The model under review builds one solid part; all positions refer to its coordinate system, in mm. A direction names the side the tool comes from. Give positions to 0.01 mm unless a question says otherwise; leave off trailing zeros. Write each loop counter-clockwise with the first axis right and the second up, starting at its lowest first coordinate (ties: lowest second). Pieces come first, ordered by that corner, then holes. Notation, with made-up numbers: M 83.25,-18.75 L 99.25,-18.75 A37 ccw 99.25,17.25 Z; hole C 21,63.25 d7. An arc over 180 degrees is marked long. Write each question's results on one line, items separated by ' | '. Start each with the question number.
from build123d import *

# Parameters (mm, degrees)
CROQUIS1_W                 = 2.5
CROQUIS1_H                 = 13.5
SALIENTE_EXTRUIR1_DEPTH    = 4.5
CORTAR_EXTRUIR4_DEPTH      = 10
CORTAR_EXTRUIR4_DEPTH_BACK = 23.169799277
CROQUIS7_R                 = 1.125
REDONDEO3_R                = 1


with BuildPart() as part:
    # Croquis1 → Saliente-Extruir1 (new body)
    with BuildSketch(Plane(origin=(0, 0, 0), x_dir=(1, 0, 0), z_dir=(0, 1, 0))):
        with BuildLine():
            Line((-2, -10), (2, -10))
            ThreePointArc((2, -10), (4.121320344, -9.121320344), (5, -7))
            Line((5, -7), (11, -7))
            Line((11, -7), (11, -3))
            Line((11, -3), (5, -3))
            Line((5, -3), (5, 3))
            Line((5, 3), (11, 3))
            Line((11, 3), (11, 7))
            Line((11, 7), (5, 7))
            ThreePointArc((5, 7), (4.121320344, 9.121320344), (2, 10))
            Line((2, 10), (-2, 10))
            ThreePointArc((-2, 10), (-4.121320344, 9.121320344), (-5, 7))
            Line((-5, 7), (-17, 7))
            Line((-17, 7), (-17, 3))
            Line((-17, 3), (-5, 3))
            Line((-5, 3), (-5, -3))
            Line((-5, -3), (-17, -3))
            Line((-17, -3), (-17, -7))
            Line((-17, -7), (-5, -7))
            ThreePointArc((-5, -7), (-4.121320344, -9.121320344), (-2, -10))
        make_face()
        Rectangle(CROQUIS1_W, CROQUIS1_H, mode=Mode.SUBTRACT)
    extrude(amount=SALIENTE_EXTRUIR1_DEPTH)

    # Croquis7 → Cortar-Extruir4 (cut, two sides: drawn at the far end of the back side and taken through both)
    with BuildSketch(Plane.XY.offset(3.5).offset(-CORTAR_EXTRUIR4_DEPTH_BACK)):
        with Locations(Location((-14.5, 2.25, 0), (0, 0, 180))):
            Circle(CROQUIS7_R)
        with Locations(Location((8.5, 2.25, 0), (0, 0, 180))):
            Circle(CROQUIS7_R)
        with Locations(Location((-7.5, 2.25, 0), (0, 0, 180))):
            Circle(CROQUIS7_R)
    extrude(amount=CORTAR_EXTRUIR4_DEPTH + CORTAR_EXTRUIR4_DEPTH_BACK, mode=Mode.SUBTRACT)

    # Redondeo3
    redondeo3_edges = [part.edges().sort_by_distance(p)[0] for p in [
        (5, 0, 0),
        (5, 4.5, 0),
    ]]
    fillet(redondeo3_edges, radius=REDONDEO3_R)


solid = part.part
(1) Draft analysis for pull direction Z (two halves, no side actions). For faces 1 (the cylindrical face through (7.427, 1.912, 4.972)), 2 (the flat face through (-11, 2, -7)), 3 (the flat face through (0, 2, -6.75)), 4 (the flat face through (-11, 2, 7)), state which applies: pulls with the +Z half, pulls with the -Z half, needs draft (parallel to the pull), parting line crosses it, or undercut.
(2) Add section C-C (x = 8.5). State the section outline as (y, z) points (3 decimals), then the cut area to 3 significant figures.
(3) Clearance check with flat-ended pins moving along their axes: P1, Ø1, axis at x = -6.5, z = 2, coming from the -Y side; P2, Ø2, axis at y = 3, z = 1, coming from the -X side; P3, Ø2, axis at x = -13, y = 3, coming from the -Z side; P4, Ø1.3, axis at y = 2.5, z = 0.5, coming from the +X side. State where each tip first meets the part, or that it passes through.
(4) Add section D-D (z = 5). State the section outline as (x, y) points (3 decimals), then the cut area to 3 significant figures.
(5) Wall thickness on L1, parallel to Z at x = -11, y = 1.8; L2, parallel to Y at x = -14.5, z = -5.65 (3 decimals); L3, parallel to X at y = 1.5, z = 5.75: over which ranges is each line inside the solid? List them lowest first.
(6) Machinability: for faces 5 (the cylindrical face through (4.699, 4.215, -0.042)), 6 (the flat face through (0, 2, 6.75)), 7 (the flat face through (7, 2, -7)), which of the approach directions +Z, -Z, +X, -X, +Y, -Y give a long, thin tool a straight path to every point of the face, cutting with its end or side? Answer none if there is none.
(7) Add section A-A (x = 5.5). State the section outline as (y, z) points.
(8) Add section B-B (z = 1). State the section outline as (x, y) points, then the cut area to 3 significant figures.
Calculated:
1) face 1: needs draft | face 2: pulls with the -Z half | face 3: undercut | face 4: pulls with the +Z half
2) outline: M 0,-7 L 1.125,-7 L 1.125,-3 L 0,-3 Z; M 0,3 L 1.125,3 L 1.125,7 L 0,7 Z; M 3.375,-7 L 4.5,-7 L 4.5,-3 L 3.375,-3 Z; M 3.375,3 L 4.5,3 L 4.5,7 L 3.375,7 Z | area: 18.0 mm²
3) P1: passes through | P2: stops at x = -5 | P3: stops at z = -7 | P4: stops at x = 5
4) outline: M -17,0 L -1.25,0 L -1.25,4.5 L -17,4.5 Z; M 1.25,0 L 11,0 L 11,4.5 L 1.25,4.5 Z; hole C -14.5,2.25 d2.25; hole C -7.5,2.25 d2.25; hole C 8.5,2.25 d2.25 | area: 103 mm²
5) L1: z = -7 to -3, 3 to 7 | L2: y = 0 to 1.125, 3.375 to 4.5 | L3: x = -17 to -15.34, -13.66 to -8.34, -6.66 to -1.25, 1.25 to 7.66, 9.34 to 11
6) face 5: +X, +Y | face 6: +Y, -Y | face 7: -Z, +X, +Y, -Y
7) outline: M 0,-7 L 4.5,-7 L 4.5,-3 L 0,-3 Z; M 0,3 L 4.5,3 L 4.5,7 L 0,7 Z
8) outline: M -5,0 L -1.25,0 L -1.25,4.5 L -5,4.5 Z; M 1.25,0 L 4,0 A1 ccw 5,1 L 5,3.5 A1 ccw 4,4.5 L 1.25,4.5 Z | area: 33.3 mm²
